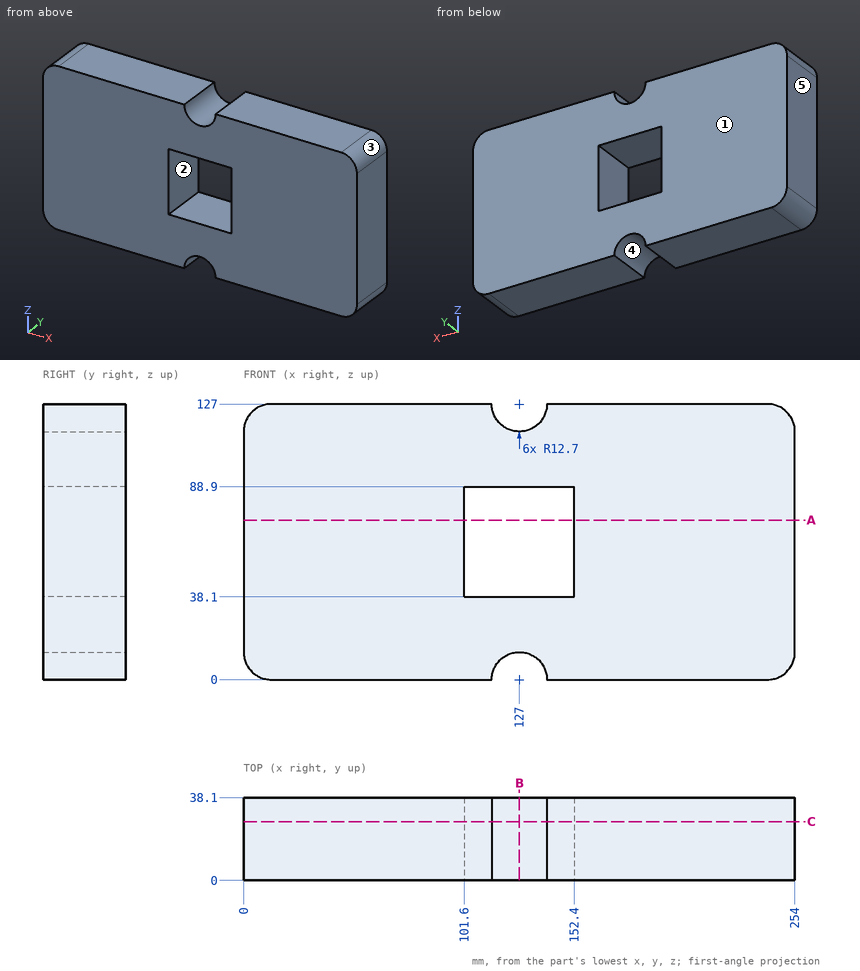
Print and shaded views of the part. All mm, measured from the part's lowest x, y and z. A direction names the side the tool comes from. Give positions to 0.01 mm unless a question says otherwise; leave off trailing zeros. Order: outer loops, then holes, each group sorted by start corner. A loop starts at its lowest first (then second) coordinate and runs counter-clockwise, first axis right, second up. Notation, with made-up numbers: (83.25, 21.25) -> (104.25, 21.25) arc R31 ccw to (104.25, 55.25) -> close; hole circle Ø10 at (37.25, 13.5). An arc over 180 degrees is marked (long way). Use CSV: the item, a comma, the result in double quotes.
1. Band-saw the part on C-C, the plane y = 27. Give the cut face in (x, z), then the cut area to 3 significant figures.
Outcome:
outline,"(0, 12.7) arc R12.7 ccw to (12.7, 0) -> (114.3, 0) arc R12.7 cw to (139.7, 0) -> (241.3, 0) arc R12.7 ccw to (254, 12.7) -> (254, 114.3) arc R12.7 ccw to (241.3, 127) -> (139.7, 127) arc R12.7 cw to (114.3, 127) -> (12.7, 127) arc R12.7 ccw to (0, 114.3) -> close; hole (101.6, 38.1) -> (152.4, 38.1) -> (152.4, 88.9) -> (101.6, 88.9) -> close"
area,"29,000 mm²"
2. Band-saw the part on B-B, the plane x = 127. Give the cut face in (y, z).
Outcome:
outline,"(0, 12.7) -> (38.1, 12.7) -> (38.1, 38.1) -> (0, 38.1) -> close; (0, 88.9) -> (38.1, 88.9) -> (38.1, 114.3) -> (0, 114.3) -> close"
3. Mould opens along X. For the marked faces 3, 4 and 5 say: +X half, -X half, draft (parallel to the pull), parting line (faces both ways), or undercut.
Outcome:
face 3,"+X half"
face 4,"undercut"
face 5,"-X half"
4. Drill centre lines: line 1 along X through (y, z) = (15, 78.5); line 2 along Z through (x, y) = (140, 18.5); line 3 along Z through (x, y) = (131.5, 2). Where is each one in solid material? Low to high. Write a range as from..to.
Outcome:
line 1,"0..101.6, 152.4..254"
line 2,"0..38.1, 88.9..127"
line 3,"11.88..38.1, 88.9..115.12"
5. Band-saw the part on A-A, the plane z = 73.5. Give the cut face in (x, y).
Outcome:
outline,"(0, 0) -> (101.6, 0) -> (101.6, 38.1) -> (0, 38.1) -> close; (152.4, 0) -> (254, 0) -> (254, 38.1) -> (152.4, 38.1) -> close"
6. 3-axis set-ups, long thin cutter, end or side, ignore diameter. For the marked faces 1 and 2: which of +Z, -Z, +X, -X, +Y, -Y reach the whole face in a straight line?
Outcome:
face 1,"+Z, -Z, +X, -X, +Y"
face 2,"+Y, -Y"
7. Drop a flat-ended pin along its axis: pin 1 (6 mm diameter, centred on x = 117, z = 83, fed in from +Y) (3 decimals). Give the stop position or say it passes through.
Outcome:
pin 1,"through"
